Design review of the part built by this model. Coordinates are the model's own, in mm. Give positions to 0.01 mm unless a question says otherwise; leave off trailing zeros. Loops run counter-clockwise (first coordinate to the right, second up) from the corner with the lowest first, then second, coordinate; pieces in that order, holes last.
Autodesk Inventor part; units mm, degrees
ref_plane "YZ Plane" through (0, 0, 0) normal (1, 0, 0) x (0, 1, 0)
ref_plane "XZ Plane" through (0, 0, 0) normal (0, 1, 0) x (-1, 0, 0)
ref_plane "XY Plane" through (0, 0, 0) normal (0, 0, 1) x (1, 0, 0)
sketch "Sketch1" plane through (0, 0, 0) normal (0, 0, 1) x (1, 0, 0)
  line L0 (-76.2, -38.1) -> (76.2, -38.1)
  line L1 (76.2, -38.1) -> (76.2, 38.1)
  line L2 (76.2, 38.1) -> (-76.2, 38.1)
  line L3 (-76.2, 38.1) -> (-76.2, -38.1)
  line L4 (-76.2, -38.1) -> (76.2, 38.1) construction
  line L5 (76.2, -38.1) -> (-76.2, 38.1) construction
  point P0 (0, 0)
  dimension "d0" = 152.4
  dimension "d1" = 76.2
extrude "Extrusion1" add sketch "Sketch1" along normal blind 6.35
sketch "Sketch2" plane through (0, 0, 6.35) normal (0, 0, 1) x (1, 0, 0)
  line L0 (63.5, 0) -> (63.5, 22.225) construction
  line L1 (63.5, 22.225) -> (63.5, -22.225) construction
  line L2 (63.5, 22.225) -> (-63.5, 22.225) construction
  line L3 (-63.5, 22.225) -> (-63.5, -22.225) construction
  line L4 (-63.5, -22.225) -> (63.5, -22.225) construction
  line L5 (63.5, -22.225) -> (63.5, 22.225) construction
  point P0 (0, 0)
  dimension "d4" = 63.5
  dimension "d7" = 127
  dimension "d16" = 44.45
  dimension "d17" = 127
  dimension "d18" = 22.225
  dimension "d19" = 63.5
hole "Hole1" at (-63.5, 22.225, 6.35) at (-63.5, -22.225, 6.35) at (63.5, -22.225, 6.35) at (63.5, 22.225, 6.35) direction (0, 0, -1) diameter 7.9375 depth 19.05 tip angle 118
properties part number "Arm Support Plate"
Q1. Draft analysis for pull direction Y (two halves, no side actions). For faces 1 (the face through (-67.435, 22.742, 3.131)), 2 (the face through (1, 38.1, 3)), 3 (the face through (-76.2, 1, 3)), 4 (the face through (59.565, -21.708, 3.131)), state which applies: pulls with the +Y half, pulls with the -Y half, needs draft (parallel to the pull), parting line crosses it, or undercut.
Results:
face 1: undercut
face 2: pulls with the +Y half
face 3: needs draft
face 4: undercut
Q2. Take a section at A-A (x = 63.5). Give the boundary of the cut face in (y, z).
Results:
outline: (-38.1, 0) - (-26.19, 0) - (-26.19, 6.35) - (-38.1, 6.35) - close; (-18.26, 0) - (18.26, 0) - (18.26, 6.35) - (-18.26, 6.35) - close; (26.19, 0) - (38.1, 0) - (38.1, 6.35) - (26.19, 6.35) - close
Q3. Take a section at C-C (x = -65.5). Give the boundary of the cut face in (y, z), plus the area to 3 significant figures.
Results:
outline: (-38.1, 0) - (-25.65, 0) - (-25.65, 6.35) - (-38.1, 6.35) - close; (-18.8, 0) - (18.8, 0) - (18.8, 6.35) - (-18.8, 6.35) - close; (25.65, 0) - (38.1, 0) - (38.1, 6.35) - (25.65, 6.35) - close
area: 397 mm2
Q4. Wall thickness on line 1 (Y direction, x = -63.5, z = 1.75); line 2 (Y direction, x = 66.5, z = 2.25); line 3 (X direction, y = -25.5, z = 2.25): over which ranges is each line inside the solid? List them lowest first.
Results:
line 1: y = -38.1 to -26.19, -18.26 to 18.26, 26.19 to 38.1
line 2: y = -38.1 to -24.82, -19.63 to 19.63, 24.82 to 38.1
line 3: x = -76.2 to -65.74, -61.26 to 61.26, 65.74 to 76.2
Q5. Take a section at B-B (z = 3.5). Give the boundary of the cut face in (x, y) (1 decimal).
Results:
outline: (-76.2, -38.1) - (76.2, -38.1) - (76.2, 38.1) - (-76.2, 38.1) - close; hole circle Ø7.9 at (-63.5, -22.2); hole circle Ø7.9 at (-63.5, 22.2); hole circle Ø7.9 at (63.5, -22.2); hole circle Ø7.9 at (63.5, 22.2)
